Check sheet for the modelled part. Datum: model origin and axes. Units: mm. Face numbers are marked on the shaded views. A direction names the side the tool comes from. Round coordinates to 2 decimals unless told otherwise and drop trailing zeros. Loops run counter-clockwise (first coordinate to the right, second up) from the corner with the lowest first, then second, coordinate; pieces in that order, holes last. Notation, with made-up numbers: (-21, 81) -> (36, 81) arc R20 ccw to (36, 109) -> close; hole circle Ø8 at (49.5, 68). An arc over 180 degrees is marked (long way). Return JSON: item names as keys, results as strings.
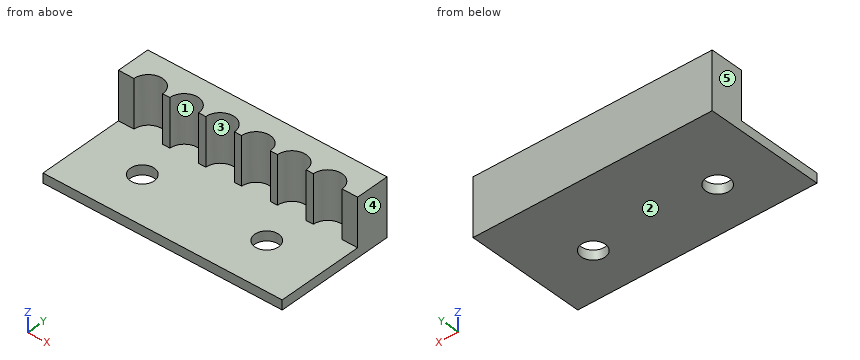
Autodesk Fusion 360 part; units mm, degrees
sketch "Sketch1" plane through (0, 0, 0) normal (0, 0, 1) x (1, 0, 0)
  line L0 (0, 0) -> (50, 0)
  line L1 (50, 0) -> (50, 25)
  line L2 (50, 25) -> (0, 25)
  line L3 (0, 25) -> (0, 0)
  circle A0 centre (12, 10) radius 2.5
  circle A1 centre (38, 10) radius 2.5
  line L4 (0, 25) -> (50, 25)
  line L5 (50, 25) -> (50, 18)
  line L6 (50, 18) -> (0, 18)
  line L7 (0, 18) -> (0, 25)
  circle A2 centre (6.25, 18) radius 3
  circle A3 centre (13.75, 18) radius 3
  circle A4 centre (21.25, 18) radius 3
  circle A5 centre (28.75, 18) radius 3
  circle A6 centre (36.25, 18) radius 3
  circle A7 centre (43.75, 18) radius 3
  dimension "d1" = 50
  dimension "d2" = 25
  dimension "d3" = 5
  dimension "d4" = 12
  dimension "d5" = 5
  dimension "d6" = 12
  dimension "d7" = 7
  dimension "d8" = 6
  dimension "d9" = 6
  dimension "d10" = 7.5
  dimension "d11" = 6
  dimension "d12" = 6
  dimension "d13" = 6
  dimension "d14" = 6
  dimension "d15" = 7.5
  dimension "d16" = 7.5
  dimension "d17" = 7.5
  dimension "d18" = 7.5
  dimension "d19" = 6.25
  dimension "d20" = 10
  dimension "d21" = 10
extrude "Extrude1" add sketch "Sketch1" along normal blind 2
extrude "Extrude2" add sketch "Sketch1" along normal blind 12 contours L1 L2 L3 L4 L5 L6 L7 A2 A3 A4 A5 A6 A7
Q1. Tool access check on the marked faces 1 and 2. Record the directions out of +Z, -Z, +X, -X, +Y, -Y that give a thin tool (end or side, any length) a straight path to the whole face; none if there is none.
Results list:
{"face 1": "+Z, -Y", "face 2": "-Z, +X, -X, +Y, -Y"}
Q2. Section check B-B (x = 13.75). Record the boundary of the cut face in (y, z), then the cut area to 3 significant figures.
Results list:
{"outline": "(0, 0) -> (8.21, 0) -> (8.21, 2) -> (0, 2) -> close; (11.79, 0) -> (25, 0) -> (25, 12) -> (21, 12) -> (21, 2) -> (11.79, 2) -> close", "area": "82.9 mm^2"}
Q3. Section check D-D (x = 21.25). Record the boundary of the cut face in (y, z).
Results list:
{"outline": "(0, 0) -> (25, 0) -> (25, 12) -> (21, 12) -> (21, 2) -> (0, 2) -> close"}
Q4. Draft check along X on the marked faces 3, 4 and 5. Enter one of: released by +X, released by -X, zero draft, split by the parting line, or undercut.
Results list:
{"face 3": "undercut", "face 4": "released by +X", "face 5": "released by -X"}
Q5. Section check A-A (y = 10). Record the boundary of the cut face in (x, z).
Results list:
{"outline": "(0, 0) -> (9.5, 0) -> (9.5, 2) -> (0, 2) -> close; (14.5, 0) -> (35.5, 0) -> (35.5, 2) -> (14.5, 2) -> close; (40.5, 0) -> (50, 0) -> (50, 2) -> (40.5, 2) -> close"}
Q6. Material ranges on line 1 (Y direction, x = 12, z = 0.95); line 2 (Z direction, x = 29, y = 8); line 3 (Y direction, x = 36.5, z = 4.25), recorded low to high.
Results list:
{"line 1": "0 to 7.5, 12.5 to 25", "line 2": "0 to 2", "line 3": "20.99 to 25"}
Q7. Go/stop test with flat-tipped pins: pin 1 (1.6 mm diameter, centred on x = 25.5, z = 9, fed in from -Y); pin 2 (6 mm diameter, centred on x = 12, y = 10, fed in from +Z). Record where each tip stops, or that it passes through.
Results list:
{"pin 1": "y = 18", "pin 2": "z = 2"}
Q8. Section check C-C (z = 7.25). Record the boundary of the cut face in (x, y).
Results list:
{"outline": "(0, 18) -> (3.25, 18) arc R3 cw to (9.25, 18) -> (10.75, 18) arc R3 cw to (16.75, 18) -> (18.25, 18) arc R3 cw to (24.25, 18) -> (25.75, 18) arc R3 cw to (31.75, 18) -> (33.25, 18) arc R3 cw to (39.25, 18) -> (40.75, 18) arc R3 cw to (46.75, 18) -> (50, 18) -> (50, 25) -> (0, 25) -> close"}
